Here's the drawing with two shaded views (mm, measured from the low corner). I have some questions. A direction names the side the tool comes from. Round coordinates to 2 decimals unless told otherwise and drop trailing zeros. Loops run counter-clockwise (first coordinate to the right, second up) from the corner with the lowest first, then second, coordinate; pieces in that order, holes last.
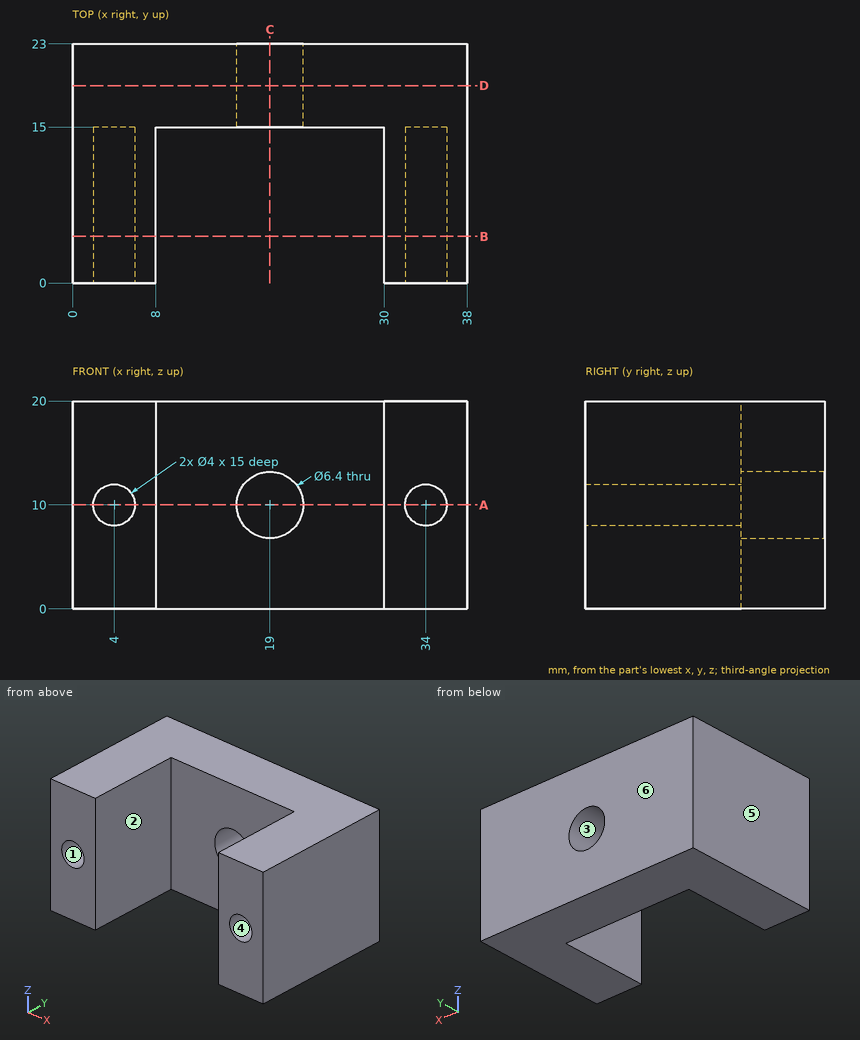
(1) If we section it at A-A, the plane z = 10: List the corners of the cut face in (x, y) for me.
Worked answers:
outline: (0, 0) - (2, 0) - (2, 15) - (6, 15) - (6, 0) - (8, 0) - (8, 15) - (15.8, 15) - (15.8, 23) - (0, 23) - close; (22.2, 15) - (30, 15) - (30, 0) - (32, 0) - (32, 15) - (36, 15) - (36, 0) - (38, 0) - (38, 23) - (22.2, 23) - close
(2) If we section it at C-C, the plane x = 19: List the corners of the cut face in (y, z) for me.
Worked answers:
outline: (15, 0) - (23, 0) - (23, 6.8) - (15, 6.8) - close; (15, 13.2) - (23, 13.2) - (23, 20) - (15, 20) - close
(3) For the marked faces 1, 2 and 3, which set-ups out of +Z, -Z, +X, -X, +Y, -Y let a thin tool reach every point of the face, with its end or its side?
Worked answers:
face 1: -Y
face 2: +Z, -Z, -Y
face 3: +Y, -Y
(4) If we mould it in two halves opening along X, with no side actions, what happens to the marked faces 4, 5 and 6? For each: released by +X, released by -X, zero draft, split by the parting line, or undercut.
Worked answers:
face 4: undercut
face 5: released by -X
face 6: zero draft
(5) If I drill on line 1 (X direction, y = 5.25, z = 10); line 2 (X direction, y = 14.5, z = 17.25); line 3 (X direction, y = 20.25, z = 10), over which ranges is the centre line in solid material (lowest first)?
Worked answers:
line 1: x = 0 to 2, 6 to 8, 30 to 32, 36 to 38
line 2: x = 0 to 8, 30 to 38
line 3: x = 0 to 15.8, 22.2 to 38
(6) Will these pins go through, and if not, where does the flat tip stop? P1, Ø5, axis at x = 27, y = 20.5, coming from the -Z side; P2, Ø5, axis at x = 19, z = 10, coming from the -Y side; P3, Ø2, axis at x = 26, z = 11, coming from the -Y side.
Worked answers:
P1: stops at z = 0
P2: passes through
P3: stops at y = 15
(7) If we section it at D-D, the plane y = 19: List the corners of the cut face in (x, z) for me, then the cut area to 3 significant figures.
Worked answers:
outline: (0, 0) - (38, 0) - (38, 20) - (0, 20) - close; hole circle Ø6.4 at (19, 10)
area: 728 mm2
(8) If we section it at B-B, the plane y = 4.5: List the corners of the cut face in (x, z) for me, then the cut area to 3 significant figures.
Worked answers:
outline: (0, 0) - (8, 0) - (8, 20) - (0, 20) - close; (30, 0) - (38, 0) - (38, 20) - (30, 20) - close; hole circle Ø4 at (4, 10); hole circle Ø4 at (34, 10)
area: 295 mm2
